```python
from build123d import *

# Parameters (mm, degrees)
BOSS_EXTRUDE1_DEPTH = 9.525
CHAMFER1_SIZE       = 50
FILLET2_R           = 5


with BuildPart() as part:
    # Sketch1 → Boss-Extrude1 (new body)
    with BuildSketch(Plane(origin=(0, 0, 0), x_dir=(1, 0, 0), z_dir=(0, 1, 0))):
        with BuildLine():
            Line((-840, 332.5), (-840, 95.5))
            Line((-840, 95.5), (-364, 95.5))
            Line((-364, 95.5), (-364, -95.5))
            Line((-364, -95.5), (-840, -95.5))
            Line((-840, -95.5), (-840, -332.5))
            Line((-840, -332.5), (-825, -332.5))
            ThreePointArc((-825, -332.5), (-803.786796564, -341.286796564), (-795, -362.5))
            Line((-795, -362.5), (795, -362.5))
            ThreePointArc((795, -362.5), (803.786796564, -341.286796564), (825, -332.5))
            Line((825, -332.5), (840, -332.5))
            Line((840, -332.5), (840, -95.5))
            Line((840, -95.5), (364, -95.5))
            Line((364, -95.5), (364, 95.5))
            Line((364, 95.5), (840, 95.5))
            Line((840, 95.5), (840, 332.5))
            Line((840, 332.5), (825, 332.5))
            ThreePointArc((825, 332.5), (803.786796564, 341.286796564), (795, 362.5))
            Line((795, 362.5), (-795, 362.5))
            ThreePointArc((-795, 362.5), (-803.786796564, 341.286796564), (-825, 332.5))
            Line((-825, 332.5), (-840, 332.5))
        make_face()
    extrude(amount=BOSS_EXTRUDE1_DEPTH)

    # Chamfer1
    chamfer1_edges = [part.edges().sort_by_distance(p)[0] for p in [
        (-364, 4.7625, 95.5),
        (-364, 4.7625, -95.5),
        (364, 4.7625, -95.5),
        (364, 4.7625, 95.5),
    ]]
    chamfer(chamfer1_edges, length=CHAMFER1_SIZE)

    # Fillet2
    fillet2_edges = [part.edges().sort_by_distance(p)[0] for p in [
        (364, 4.7625, -45.5),
        (364, 4.7625, 45.5),
        (414, 4.7625, 95.5),
        (414, 4.7625, -95.5),
        (-414, 4.7625, 95.5),
        (-364, 4.7625, -45.5),
        (-364, 4.7625, 45.5),
        (-414, 4.7625, -95.5),
    ]]
    fillet(fillet2_edges, radius=FILLET2_R)


solid = part.part
```
Work out the finished part from the listing and answer in its coordinate system (mm). A direction names the side the tool comes from. Give positions to 0.01 mm unless a question says otherwise; leave off trailing zeros. Loops run counter-clockwise (first coordinate to the right, second up) from the corner with the lowest first, then second, coordinate; pieces in that order, holes last. Notation, with made-up numbers: (71.25, 36) - (123.25, 36) arc R21 cw to (123.25, 61) - close; hole circle Ø1 at (11, 30.25). An arc over 180 degrees is marked (long way). One line per question, with ' | ' between items.
(1) Straight lines are drawn through the part: probe 1 along Z at (x, y) = (657, 1); probe 2 along X at (y, z) = (3, 5.5). For each, find the intervals that lie inside material, in ascending order.
Recorded:
probe 1: z = -362.5 to -95.5, 95.5 to 362.5 | probe 2: x = -364 to 364
(2) A tool of negligible diameter and unlimited length cuts with its end or side. For faces 1 (the face through (-804.021, 4.696, 341.055)), 2 (the face through (-388.7, 4.7, -70.2)), 3 (the face through (389.3, 4.7, -70.8)), from which of +Z, -Z, +X, -X, +Y, -Y can it reach the whole face along a straight path? Write none if from no direction.
Recorded:
face 1: +Z, -X, +Y, -Y | face 2: -X, +Y, -Y | face 3: +X, +Y, -Y
(3) The part is cut by section A-A (x = -553.5). Write down the section's boundary in (y, z) (3 decimals), then the cut area to 3 significant figures.
Recorded:
outline: (0, -362.5) - (9.525, -362.5) - (9.525, -95.5) - (0, -95.5) - close; (0, 95.5) - (9.525, 95.5) - (9.525, 362.5) - (0, 362.5) - close | area: 5,090 mm²
(4) The part is cut by section C-C (z = -76). Write down the section's boundary in (x, y) (3 decimals).
Recorded:
outline: (-394.5, 0) - (394.5, 0) - (394.5, 9.525) - (-394.5, 9.525) - close
(5) Each of these flat-tipped pins is pushed along its axis until it touches: pin 1 Ø3 at (x, y) = (-829.5, 3) entering from +Z; pin 2 Ø5 at (y, z) = (3.5, -6.5) entering from -X; pin 3 Ø3 at (x, y) = (-832, 4) entering from -Z. Where does it stop, or does it pass through?
Recorded:
pin 1: stops at z = 332.5 | pin 2: stops at x = -364 | pin 3: stops at z = -332.5
